```python
from build123d import *

# Parameters (mm, degrees)
F0_R      = 15
F2_R      = 15.875
F4_R      = 5
F6_R      = 5.25
F7_FACE_R = 5.25
F9_R      = 4.25
F11_R     = 2
F12_DEPTH = 25.0010001
F13_R     = 1.5
F15_R     = 2


with BuildPart() as f3:
    # F0 (on Top) → F3 section 0
    with BuildSketch(Plane.XY):
        Circle(F0_R)
    # F2 (on offset) → F3 section 1
    with BuildSketch(Plane.XY.offset(18.5)):
        Circle(F2_R)
    loft()

    # F4 (on face) → F7 section 0
    with BuildSketch(Plane.XY.offset(18.5)):
        Circle(F4_R)
    # F6 (on offset) → F7 section 1
    with BuildSketch(Plane.XY.offset(22.5)):
        Circle(F6_R)
    loft()

    # F7_face (on face) → F10 section 0
    with BuildSketch(Plane.XY.offset(22.5)):
        Circle(F7_FACE_R)
    # F9 (on offset) → F10 section 1
    with BuildSketch(Plane.XY.offset(25)):
        Circle(F9_R)
    loft()

    # F11 (on face) → F12 (cut, through all)
    with BuildSketch(Plane.XY.offset(25)):
        Circle(F11_R)
    extrude(amount=-F12_DEPTH, mode=Mode.SUBTRACT)

    # F13 (on Front) → F14 (revolve, cut)
    with BuildSketch(Plane.XZ):
        with Locations((-9.7052594647, 0)):
            Circle(F13_R)
    revolve(axis=Axis((0, 0, 7.5749068208), (0, 0, -1)), mode=Mode.SUBTRACT)

    # F15
    f15_edges = [f3.edges().sort_by_distance(p)[0] for p in [
        (-15, 0, 0),
    ]]
    fillet(f15_edges, radius=F15_R)


solid = f3.part
```
Input: part model. Units: mm. Frame: model coordinates. Give positions to 0.01 mm unless a question says otherwise; leave off trailing zeros. Order: outer loops, then holes, each group sorted by start corner. A loop starts at its lowest first (then second) coordinate and runs counter-clockwise, first axis right, second up. Notation, with made-up numbers: M 82,14 L 122,14 A11 ccw 122,32 Z; hole C 51,-26.75 d1. An arc over 180 degrees is marked long. Return JSON: item names as keys, results as strings.
1) Line query: L1, parallel to Z at x = 0.5, y = 12; L2, parallel to Y at x = -6.5, z = 1; L3, parallel to Y at x = 0, z = 13.75. Output: solid intervals per line, ascending. Write a range as [from, to].
Taken from the geometry:
{"L1": "z = [0, 18.5]", "L2": "y = [-13.32, -8.65], [-5.61, 5.61], [8.65, 13.32]", "L3": "y = [-15.65, -2], [2, 15.65]"}
2) Section query C-C on z = 6.75. Output: boundary loops of the cut face in (x, y), and give its area (3 significant figures).
Taken from the geometry:
{"outline": "C 0,0 d30.64; hole C 0,0 d4", "area": "725 mm2"}
3) Section query A-A on x = 0. Output: boundary loops of the cut face in (y, z) (3 decimals), and give its area (3 significant figures).
Taken from the geometry:
{"outline": "M -15.875,18.5 L -15.09,1.906 A2 ccw -13.092,0 L -11.205,0 A1.5 cw -8.205,0 L -2,0 L -2,25 L -4.25,25 L -5.25,22.5 L -5,18.5 Z; M 2,0 L 8.205,0 A1.5 cw 11.205,0 L 13.092,0 A2 ccw 15.09,1.906 L 15.875,18.5 L 5,18.5 L 5.25,22.5 L 4.25,25 L 2,25 Z", "area": "527 mm2"}
4) Mould query, pull axis Y, two halves, no side actions, for faces 1 (the face through (-4.05, -3.1, 20.08)), 2 (the face through (0, -2, 13)), 3 (the face through (-4, 4, 18.5)). Classes: released by +Y, released by -Y, zero draft, split by the parting line, or undercut.
Taken from the geometry:
{"face 1": "split by the parting line", "face 2": "undercut", "face 3": "zero draft"}
5) Section query B-B on z = 16. Output: boundary loops of the cut face in (x, y).
Taken from the geometry:
{"outline": "C 0,0 d31.51; hole C 0,0 d4"}
6) Contact query for flat-ended pins moving along their axis: pin 1 (1.5 mm diameter, centred on x = 10, z = 10.5, fed in from +Y); pin 2 (3 mm diameter, centred on x = 0, y = 0, fed in from +Z); pin 3 (3 mm diameter, centred on y = -2.5, z = 5, fed in from +X); pin 4 (10 mm diameter, centred on x = 6, z = 9, fed in from -Y). Output: stop coordinate, or through.
Taken from the geometry:
{"pin 1": "stops at y = 12.43", "pin 2": "passes through", "pin 3": "stops at x = 15.22", "pin 4": "stops at y = -15.46"}
